Job drawing, mm, ordinate dimensions from the low corner. One solid piece. Coordinates: 2 decimals unless noted, no trailing zeros. Order: outer loops, then holes, each group sorted by start corner. A loop starts at its lowest first (then second) coordinate and runs counter-clockwise, first axis right, second up. Notation, with made-up numbers: (-33.75, 89) - (-14.75, 89) arc R25 ccw to (-14.75, 107) - close; hole circle Ø2 at (8.5, 17.5). An arc over 180 degrees is marked (long way). Use one line per item in the form item = value.
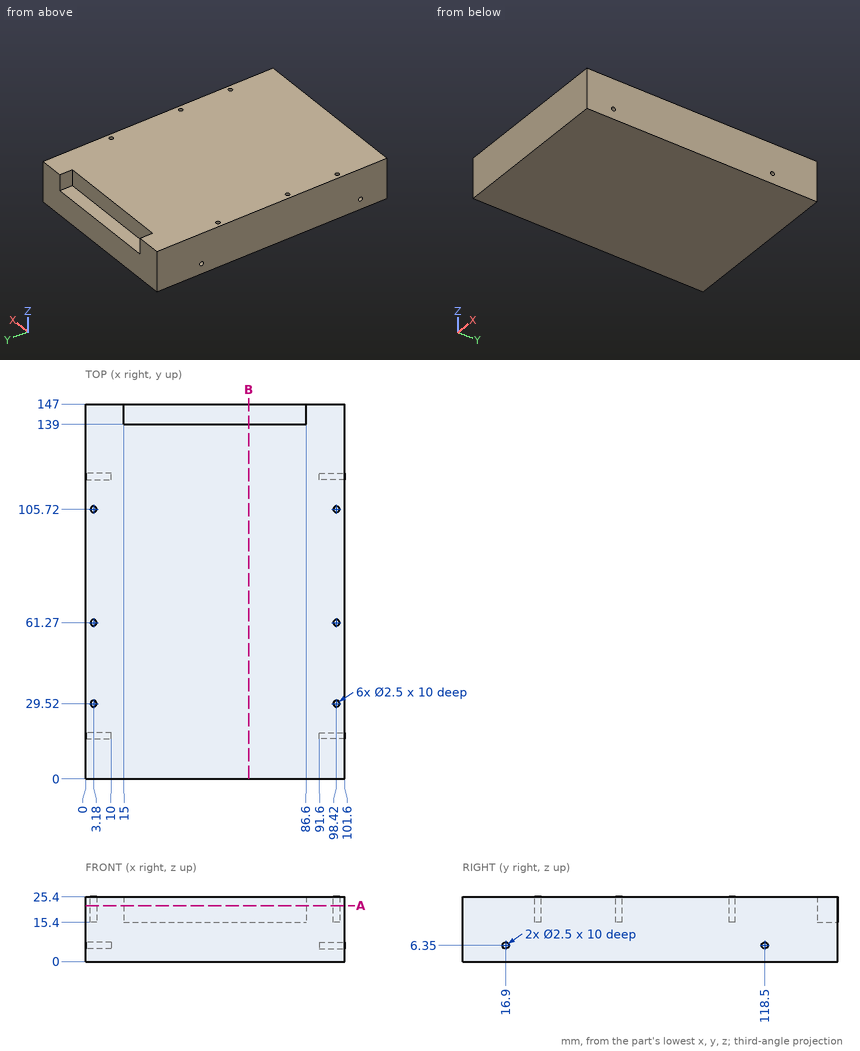
Item 1: Drill centre lines: line 1 (Y direction, x = 98.42, z = 19); line 2 (X direction, y = 105.72, z = 20.5); line 3 (Y direction, x = 67.5, z = 22.5). Where is each one in solid material? Low to high. Write a range as [from, to].
Derived:
line_1 = [0, 28.27], [30.77, 60.02], [62.52, 104.47], [106.97, 147]
line_2 = [0, 1.93], [4.43, 97.17], [99.67, 101.6]
line_3 = [0, 139]
Item 2: Cut at B-B, the plane x = 64. Write the cut outline in (y, z).
Derived:
outline = (0, 0) - (147, 0) - (147, 15.4) - (139, 15.4) - (139, 25.4) - (0, 25.4) - close
Item 3: Cut at A-A, the plane z = 22. Write the cut outline in (x, y), plus the area to 3 significant figures.
Derived:
outline = (0, 0) - (101.6, 0) - (101.6, 147) - (86.6, 147) - (86.6, 139) - (15, 139) - (15, 147) - (0, 147) - close; hole circle Ø2.5 at (3.18, 29.52); hole circle Ø2.5 at (3.18, 61.27); hole circle Ø2.5 at (3.18, 105.72); hole circle Ø2.5 at (98.42, 29.52); hole circle Ø2.5 at (98.42, 61.27); hole circle Ø2.5 at (98.42, 105.72)
area = 14,300 mm²
Item 4: Drop flat-ended pins along their axis: pin 1 (0.8 mm diameter, centred on y = 118.5, z = 7, fed in from -X); pin 2 (0.8 mm diameter, centred on x = 98, y = 29.5, fed in from +Z); pin 3 (1.5 mm diameter, centred on y = 118.5, z = 6.35, fed in from +X). Give the stop position or say it passes through.
Derived:
pin_1 = 10
pin_2 = 15.4
pin_3 = 91.6
